Read the model definition and answer for the solid it produces. Units are mm, in the model's axes. Coordinates: 2 decimals unless noted, no trailing zeros. Loops run counter-clockwise (first coordinate to the right, second up) from the corner with the lowest first, then second, coordinate; pieces in that order, holes last. Notation, with made-up numbers: M -30,-3.75 L 13,-3.75 A23 cw 13,12.25 Z; hole C -23,30 d8. An arc over 180 degrees is marked long. One line per item, written item: value. Start each with the question number.
```python
from build123d import *

# Parameters (mm, degrees)
F1_DEPTH = 3
F2_R     = 1


with BuildPart() as f1:
    # F0 (on Top) → F1 (new body)
    with BuildSketch(Plane.XY):
        with BuildLine():
            ThreePointArc((20, 4.5), (19.12132, 6.62132), (17, 7.5))
            Line((17, 7.5), (-17, 7.5))
            ThreePointArc((-17, 7.5), (-19.12132, 6.62132), (-20, 4.5))
            Line((-20, 4.5), (-20, -4.5))
            ThreePointArc((-20, -4.5), (-19.12132, -6.62132), (-17, -7.5))
            Line((-17, -7.5), (17, -7.5))
            ThreePointArc((17, -7.5), (19.12132, -6.62132), (20, -4.5))
            Line((20, -4.5), (20, 4.5))
        make_face()
    extrude(amount=-F1_DEPTH)

    # F2
    f2_edges = [f1.edges().sort_by_distance(p)[0] for p in [
        (19.12132, -6.62132, 0),
        (20, 0, 0),
        (19.12132, 6.62132, 0),
        (0, 7.5, 0),
        (-19.12132, 6.62132, 0),
        (-20, 0, 0),
        (-19.12132, -6.62132, 0),
        (0, -7.5, 0),
        (19.12132, -6.62132, -3),
        (20, 0, -3),
        (19.12132, 6.62132, -3),
        (0, 7.5, -3),
        (-19.12132, 6.62132, -3),
        (-20, 0, -3),
        (-19.12132, -6.62132, -3),
        (0, -7.5, -3),
    ]]
    fillet(f2_edges, radius=F2_R)


solid = f1.part
```
1) Consider line 1 along Z through (x, y) = (5, -7); line 2 along X through (y, z) = (7.25, -1.25); line 3 along X through (y, z) = (-4.25, -2.15). Determine where each line is inside the solid, lowest interval first.
2) A flat-ended cylindrical pin translates along its axis: pin 1 (1.5 mm diameter, centred on y = -5.5, z = -2, fed in from +X). Find the tip coordinate at first contact, or state that the pin passes through.
3) Section B-B (z = -2.35) is taken. Determine the outline of the cut face in (x, y), then the cut area to 3 significant figures.
4) Section A-A (x = -3) is taken. Determine the outline of the cut face in (y, z), then the cut area to 3 significant figures.
Results found:
1. line 1: z = -2.87 to -0.13
1. line 2: x = -18.2 to 18.2
1. line 3: x = -19.99 to 19.99
2. pin 1: stops at x = 19.99
3. outline: M -19.94,-4.5 A2.94 ccw -17,-7.44 L 17,-7.44 A2.94 ccw 19.94,-4.5 L 19.94,4.5 A2.94 ccw 17,7.44 L -17,7.44 A2.94 ccw -19.94,4.5 Z
3. area: 586 mm²
4. outline: M -7.5,-2 A1 ccw -6.5,-3 L 6.5,-3 A1 ccw 7.5,-2 L 7.5,-1 A1 ccw 6.5,0 L -6.5,0 A1 ccw -7.5,-1 Z
4. area: 44.1 mm²
